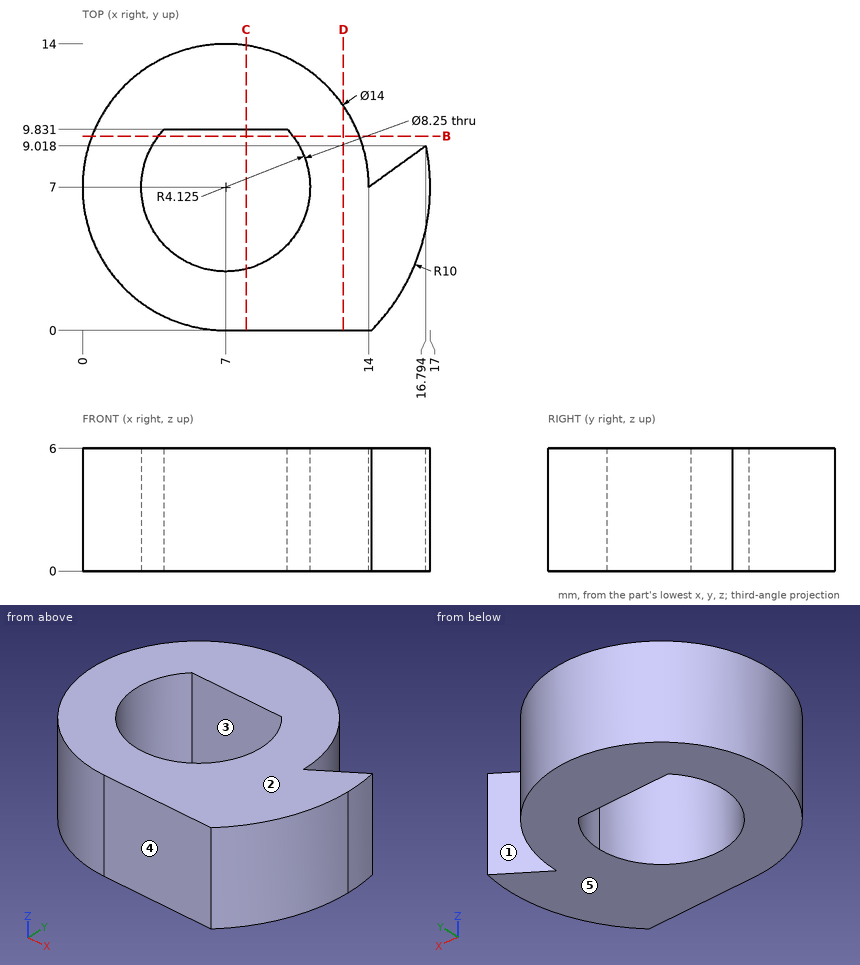
Verification items for this drawing (mm, ordinates from the low corner). A direction names the side the tool comes from. Coordinates: 2 decimals unless noted, no trailing zeros. Order: outer loops, then holes, each group sorted by start corner. A loop starts at its lowest first (then second) coordinate and runs counter-clockwise, first axis right, second up. Notation, with made-up numbers: (-19.5, -14.75) - (-12.5, -14.75) arc R22 ccw to (-12.5, -2.75) - close; hole circle Ø10 at (47.5, 78). An arc over 180 degrees is marked (long way). Use one line per item in the form item = value.
1. Scan lines: line 1 (Y direction, x = 7, z = 3.7) (1 decimal); line 2 (Y direction, x = 4.75, z = 1.65); line 3 (X direction, y = 3.5, z = 5.7) (1 decimal). Record each from-to range of solid material in increasing order.
Here are the results:
line_1 = 0 to 2.9, 9.8 to 14
line_2 = 0.37 to 3.54, 9.83 to 13.63
line_3 = 0.9 to 4.8, 9.2 to 16.4
2. Section check D-D (x = 12.75). Record the boundary of the cut face in (y, z).
Here are the results:
outline = (0, 0) - (10.99, 0) - (10.99, 6) - (0, 6) - close
3. Draft check along Y on the marked faces 3, 4 and 5. Enter one of: pulls with the +Y half, pulls with the -Y half, needs draft (parallel to the pull), parting line crosses it, or undercut.
Here are the results:
face_3 = undercut
face_4 = pulls with the -Y half
face_5 = needs draft
4. Access from +Z, -Z, +X, -X, +Y, -Y to the whole of each face (thin tool, end or side, straight path). Record for the marked faces 1 and 2.
Here are the results:
face_1 = +Z, -Z, +Y
face_2 = +Z, +X, -X, +Y, -Y
5. Section check B-B (y = 9.5). Record the boundary of the cut face in (x, z), then the cut area to 3 significant figures.
Here are the results:
outline = (0.46, 0) - (3.72, 0) - (3.72, 6) - (0.46, 6) - close; (10.28, 0) - (13.54, 0) - (13.54, 6) - (10.28, 6) - close
area = 39.1 mm²
6. Section check C-C (x = 8). Record the boundary of the cut face in (y, z).
Here are the results:
outline = (0, 0) - (3, 0) - (3, 6) - (0, 6) - close; (9.83, 0) - (13.93, 0) - (13.93, 6) - (9.83, 6) - close
7. Gauge pin test, flat ends, axial feed: pin 1 (2 mm diameter, centred on x = 10, z = 5, fed in from +Y); pin 2 (1.5 mm diameter, centred on y = 6, z = 3.5, fed in from -X). Record the tip position at first contact, or that the pin passes through.
Here are the results:
pin_1 = 13.71
pin_2 = 0
